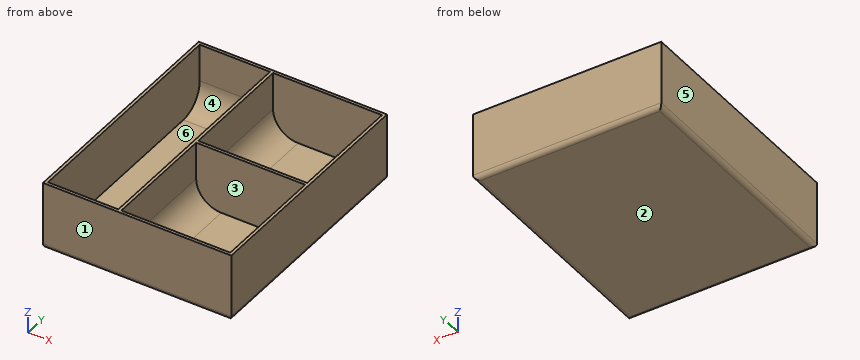
```python
from build123d import *

# Parameters (mm, degrees)
SKETCH011_W             = 75
SKETCH011_H             = 95
PAD007_DEPTH            = 1
SKETCH012_W             = 75
SKETCH012_H             = 95
SKETCH012_W_2           = 28
SKETCH012_H_2           = 92.6
SKETCH012_W_3           = 43.4
SKETCH012_H_3           = 45.7
PAD008_DEPTH            = 25
FILLET010_R             = 10
FILLET011_R             = 1.8
BODY003_PLACEMENT_ANGLE = 90


with BuildPart() as part:
    # Sketch011 → Pad007 (new body, symmetric)
    with BuildSketch(Plane.XZ):
        Rectangle(SKETCH011_W, SKETCH011_H)
    extrude(amount=PAD007_DEPTH, both=True)

    # Sketch012 → Pad008 (join)
    with BuildSketch(Plane.XZ.offset(1)):
        Rectangle(SKETCH012_W, SKETCH012_H)
        with Locations((-22.3, 0)):
            Rectangle(SKETCH012_W_2, SKETCH012_H_2, mode=Mode.SUBTRACT)
        with Locations((14.6, 23.45)):
            Rectangle(SKETCH012_W_3, SKETCH012_H_3, mode=Mode.SUBTRACT)
        with Locations((14.6, -23.45)):
            Rectangle(SKETCH012_W_3, SKETCH012_H_3, mode=Mode.SUBTRACT)
    extrude(amount=PAD008_DEPTH)

    # Fillet010
    fillet010_edges = [part.edges().sort_by_distance(p)[0] for p in [
        (36.3, -1, 23.45),
        (36.3, -1, -23.45),
        (-22.3, -1, 46.3),
        (-7.1, -1, 23.45),
        (-7.1, -1, -23.45),
        (-22.3, -1, -46.3),
    ]]
    fillet(fillet010_edges, radius=FILLET010_R)

    # Fillet011
    fillet011_edges = [part.edges().sort_by_distance(p)[0] for p in [
        (0, 1, 47.5),
        (37.5, 1, 0),
        (0, 1, -47.5),
        (-37.5, 1, 0),
    ]]
    fillet(fillet011_edges, radius=FILLET011_R)


with BuildPart() as part_1:
    # Body003 placement: moved
    add(part.part.rotate(Axis((0, 0, 0), (-1, 0, 0)), BODY003_PLACEMENT_ANGLE))


solid = part_1.part
```
Work out the finished part from the listing and answer in its coordinate system (mm). Face numbers are marked on the shaded views. A direction names the side the tool comes from. Round coordinates to 2 decimals unless told otherwise and drop trailing zeros. Loops run counter-clockwise (first coordinate to the right, second up) from the corner with the lowest first, then second, coordinate; pieces in that order, holes last.
(1) The part is cut by section C-C, the plane x = -29. Give the vertices of the cut face in (y, z), and give its area (3 significant figures).
Computed values:
outline: (-47.5, 0.8) arc R1.8 ccw to (-45.7, -1) - (45.7, -1) arc R1.8 ccw to (47.5, 0.8) - (47.5, 26) - (46.3, 26) - (46.3, 11) arc R10 cw to (36.3, 1) - (-36.3, 1) arc R10 cw to (-46.3, 11) - (-46.3, 26) - (-47.5, 26) - close
area: 292 mm2
(2) Find the intervals of material crossed by L1, parallel to Y at x = 4, z = 13.25; L2, parallel to X at y = -24, z = 18.5; L3, parallel to Y at x = -26, z = 20.75, in increasing order.
Computed values:
L1: y = -47.5 to -46.3, -0.6 to 0.6, 46.3 to 47.5
L2: x = -37.5 to -36.3, -8.3 to -7.1, 36.3 to 37.5
L3: y = -47.5 to -46.3, 46.3 to 47.5
(3) Each of these flat-tipped pins is pushed along its axis until it touches: P1, Ø1, axis at x = -9, y = 9, coming from the +Z side; P2, Ø5, axis at x = -14, y = 37.5, coming from the +Z side. Where does it stop, or does it pass through?
Computed values:
P1: stops at z = 1
P2: stops at z = 1.71
(4) The mould has two halves that part along Y. Classify the marked faces 1, 2, 3 and 4: pulls with the +Y half, pulls with the -Y half, needs draft (parallel to the pull), parting line crosses it, or undercut.
Computed values:
face 1: pulls with the -Y half
face 2: needs draft
face 3: undercut
face 4: undercut
(5) The part is cut by section D-D, the plane x = 6. Give the vertices of the cut face in (y, z).
Computed values:
outline: (-47.5, 0.8) arc R1.8 ccw to (-45.7, -1) - (45.7, -1) arc R1.8 ccw to (47.5, 0.8) - (47.5, 26) - (46.3, 26) - (46.3, 1) - (0.6, 1) - (0.6, 26) - (-0.6, 26) - (-0.6, 1) - (-46.3, 1) - (-46.3, 26) - (-47.5, 26) - close
(6) The part is cut by section A-A, the plane y = -14. Give the vertices of the cut face in (x, z).
Computed values:
outline: (-37.5, 0.8) arc R1.8 ccw to (-35.7, -1) - (35.7, -1) arc R1.8 ccw to (37.5, 0.8) - (37.5, 26) - (36.3, 26) - (36.3, 11) arc R10 cw to (26.3, 1) - (2.9, 1) arc R10 cw to (-7.1, 11) - (-7.1, 26) - (-8.3, 26) - (-8.3, 1) - (-36.3, 1) - (-36.3, 26) - (-37.5, 26) - close
(7) For the marked faces 5 and 6, determine the directions among +Z, -Z, +X, -X, +Y, -Y from which every point of the face is accessible in a straight line to the end or side of a thin tool.
Computed values:
face 5: +Z, -Z, -X, +Y, -Y
face 6: +Z
(8) The part is cut by section B-B, the plane z = 21.25. Give the vertices of the cut face in (x, y), and give its area (3 significant figures).
Computed values:
outline: (-37.5, -47.5) - (37.5, -47.5) - (37.5, 47.5) - (-37.5, 47.5) - close; hole (-36.3, -46.3) - (-8.3, -46.3) - (-8.3, 46.3) - (-36.3, 46.3) - close; hole (-7.1, -46.3) - (36.3, -46.3) - (36.3, -0.6) - (-7.1, -0.6) - close; hole (-7.1, 0.6) - (36.3, 0.6) - (36.3, 46.3) - (-7.1, 46.3) - close
area: 565 mm2
